Model file for the job. Use its own axes, mm. A direction names the side the tool comes from. Round coordinates to 2 decimals unless told otherwise and drop trailing zeros. Loops run counter-clockwise (first coordinate to the right, second up) from the corner with the lowest first, then second, coordinate; pieces in that order, holes last. Notation, with made-up numbers: M -24,49 L 30,49 A21 ccw 30,82 Z; hole C 32,63.25 d11. An arc over 180 degrees is marked long. Use a Markdown table: item, result. Add a question column.
Q1. Probe line 1 (Y direction, x = -19, z = 4); line 2 (X direction, y = 29.5, z = 9); line 3 (Y direction, x = -18, z = 27.5). List the from-to ranges inside material, lowest first. Write a range as from..to.
Q2. Cut at B-B (z = 8). Give the cut face in (x, y).
Q3. Cut at D-D (y = 29.5). Give the cut face in (x, z), plus the area to 3 significant figures.
Q4. Pin check, flat tips, straight feed: pin 1 (4.5 mm diameter, centred on x = -20.5, y = 28.5, fed in from -Z); pin 2 (8 mm diameter, centred on x = -12, y = -7, fed in from +Z); pin 3 (3 mm diameter, centred on x = -11.5, z = 40, fed in from -Y). Stop position of each tip, or through.
Q5. Tool access for faces 1 (the face through (-19, -1, 0)), 2 (the face through (-19, -30, 13)): list every direction of +Z, -Z, +X, -X, +Y, -Y with a clear straight run to the whole face (end or side of a thin tool).
Q6. Cut at C-C (z = 30.2). Give the cut face in (x, y), plus the area to 3 significant figures.
Q7. Mould opens along X. For faces 3 (the face through (-20.08, -24.62, 6.42)), 4 (the face through (-38, 8, 24)), 5 (the face through (-19, -38, 11)), 6 (the face through (-19, 29, 13)) say: +X half, -X half, draft (parallel to the pull), parting line (faces both ways), or undercut.
Q8. Cut at A-A (x = -19). Give the cut face in (y, z), plus the area to 3 significant figures.
from build123d import *

# Parameters (mm, degrees)
F1_DEPTH = 38
F2_R     = 7.5
F3_DEPTH = 38.001
F4_SIZE  = 0.5
F5_R     = 5
F6_DEPTH = 13
F7_SIZE  = 0.5


# Not quite as in the source:
# - a feature names something its author has since deleted; it is built from what else it names


with BuildPart() as f1:
    # F0 (on Right) → F1 (new body)
    with BuildSketch(Plane.YZ):
        with BuildLine():
            Line((-38, 0), (0, 0))
            Line((0, 0), (38, 0))
            Line((38, 0), (38, 22))
            ThreePointArc((38, 22), (26.8700576851, 48.8700576851), (0, 60))
            ThreePointArc((0, 60), (-26.8700576851, 48.8700576851), (-38, 22))
            Line((-38, 22), (-38, 0))
        make_face()
    extrude(amount=-F1_DEPTH)

    # F2 (on face) → F3 (cut, through all)
    with BuildSketch(Plane.YZ):
        with Locations((0, 30.2)):
            Circle(F2_R)
    extrude(amount=-F3_DEPTH, mode=Mode.SUBTRACT)

    # F4
    f4_edges = [f1.edges().sort_by_distance(p)[0] for p in [
        (0, -7.5, 30.2),
        (-19, 7.5, 30.2),
        (-38, -7.5, 30.2),
    ]]
    chamfer(f4_edges, length=F4_SIZE)

    # F5 (on face) → F6 (cut)
    with BuildSketch(Plane(origin=(0, 0, 0), x_dir=(1, 0, 0), z_dir=(0, 0, -1))):
        with Locations((-19, 29.5)):
            Circle(F5_R)
        with Locations((-19, -29.5)):
            Circle(F5_R)
    extrude(amount=-F6_DEPTH, mode=Mode.SUBTRACT)

    # F7
    f7_edges = [f1.edges().sort_by_distance(p)[0] for p in [
        (-14, -29.5, 6.5),
        (-24, -29.5, 0),
        (-24, -29.5, 13),
        (-14, 29.5, 6.5),
        (-24, 29.5, 0),
        (-24, 29.5, 13),
    ]]
    chamfer(f7_edges, length=F7_SIZE)


solid = f1.part
Checked values:
| question | item | result |
|---|---|---|
| 1 | line 1 | y = -38..-34.5, -24.5..24.5, 34.5..38 |
| 1 | line 2 | x = -38..-24, -14..0 |
| 1 | line 3 | y = -37.6..-7, 7..37.6 |
| 2 | outline | M -38,-38 L 0,-38 L 0,38 L -38,38 Z; hole C -19,-29.5 d10; hole C -19,29.5 d10 |
| 3 | outline | M -38,0 L -24.5,0 L -24,0.5 L -24,12.5 L -23.5,13 L -14.5,13 L -14,12.5 L -14,0.5 L -13.5,0 L 0,0 L 0,45.95 L -38,45.95 Z |
| 3 | area | 1,620 mm^2 |
| 4 | pin 1 | stops at z = 13 |
| 4 | pin 2 | stops at z = 59.88 |
| 4 | pin 3 | stops at y = -34.23 |
| 5 | face 1 | -Z, +X, -X, +Y, -Y |
| 5 | face 2 | -Z |
| 6 | outline | M -38,-37.1 L 0,-37.1 L 0,-8 L -0.5,-7.5 L -37.5,-7.5 L -38,-8 Z; M -38,8 L -37.5,7.5 L -0.5,7.5 L 0,8 L 0,37.1 L -38,37.1 Z |
| 6 | area | 2,250 mm^2 |
| 7 | face 3 | undercut |
| 7 | face 4 | -X half |
| 7 | face 5 | draft |
| 7 | face 6 | undercut |
| 8 | outline | M -38,0 L -35,0 L -34.5,0.5 L -34.5,12.5 L -34,13 L -25,13 L -24.5,12.5 L -24.5,0.5 L -24,0 L 24,0 L 24.5,0.5 L 24.5,12.5 L 25,13 L 34,13 L 34.5,12.5 L 34.5,0.5 L 35,0 L 38,0 L 38,22 A38 ccw -38,22 Z; hole C 0,30.2 d15 |
| 8 | area | 3,500 mm^2 |
